Job drawing, mm, ordinate dimensions from the low corner. One solid piece. A direction names the side the tool comes from. Give positions to 0.01 mm unless a question says otherwise; leave off trailing zeros. Write each loop counter-clockwise with the first axis right and the second up, starting at its lowest first coordinate (ties: lowest second). Pieces come first, ordered by that corner, then holes. Notation, with made-up numbers: M 69.25,28 L 107.25,28 A19 cw 107.25,59 Z; hole C -31,14 d8. An arc over 180 degrees is marked long. Use CSV: the item, a comma, the result in double quotes. Start each with the question number.
Item 1: Pin check, flat tips, straight feed: pin 1 (2 mm diameter, centred on y = 1, z = 185, fed in from +X); pin 2 (6 mm diameter, centred on x = 156, z = 39, fed in from +Y); pin 3 (9 mm diameter, centred on x = 169.11, z = 295.93, fed in from +Y); pin 4 (4.5 mm diameter, centred on y = 2.5, z = 178, fed in from -X). Stop position of each tip, or through.
Item 2: Drill centre lines: line 1 (X direction, y = 15.5, z = 204); line 2 (Y direction, x = 129, z = 60); line 3 (X direction, y = 5, z = 231). Where is each one in solid material? Low to high. Write a range as [from, to].
Item 3: Cut at A-A (z = 315). List the corners of the cut face in (x, y), then the cut area to 3 significant figures.
Item 4: Cut at B-B (y = 17). List the corners of the cut face in (x, z), then the cut area to 3 significant figures.
Item 5: Which spindle directions (+Z, -Z, +X, -X, +Y, -Y) get a long thin tool onto all of the face, cutting with end or side? Do the marked faces 1 and 2. Say none if no direction does.
Item 6: Cut at D-D (x = 154.5). List the corners of the cut face in (y, z), then the cut area to 3 significant figures.
Item 7: Cut at C-C (z = 122). List the corners of the cut face in (x, y).
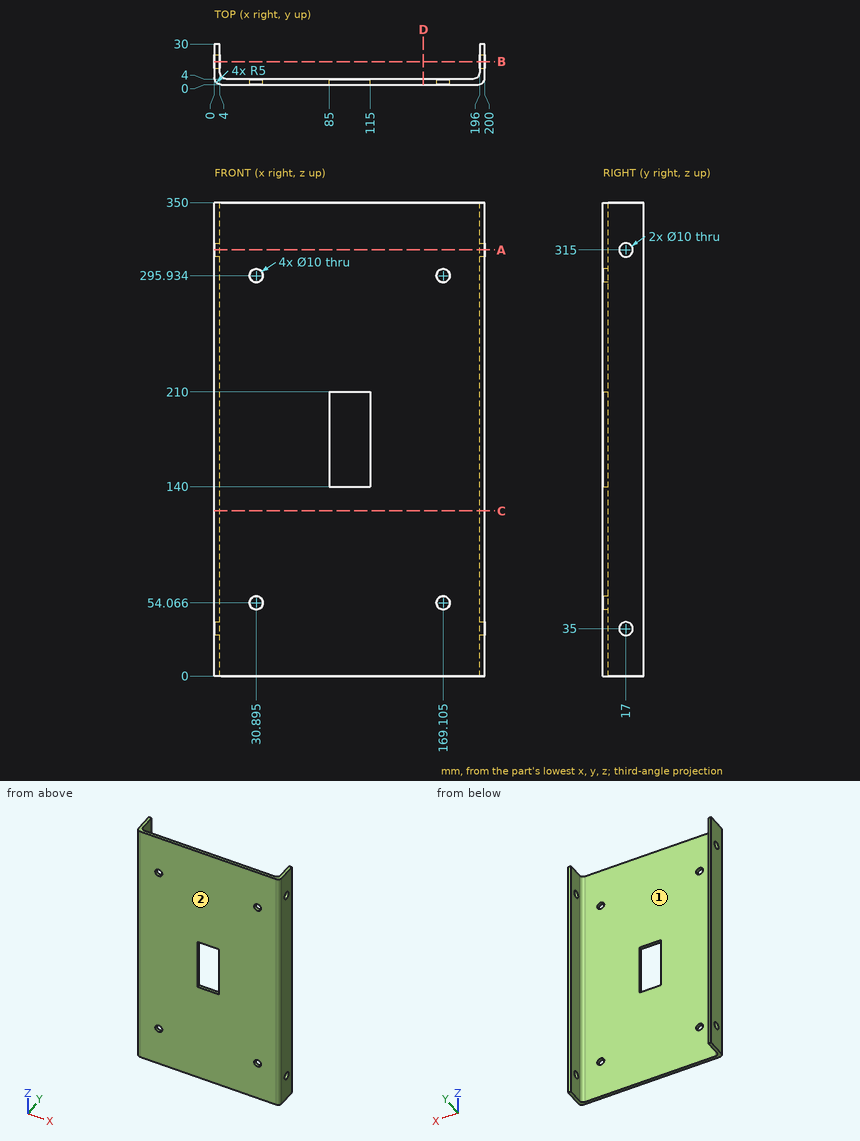
Worked answers:
1,pin 1,"stops at x = 199"
1,pin 2,"stops at y = 4"
1,pin 3,"passes through"
1,pin 4,"stops at x = 0.01"
2,line 1,"x = [0, 4], [196, 200]"
2,line 2,"y = [0, 4]"
2,line 3,"x = [0, 6], [194, 200]"
3,outline,"M 0,5 A5 ccw 5,0 L 195,0 A5 ccw 200,5 L 200,12 L 196,12 L 196,9 A5 cw 191,4 L 9,4 A5 cw 4,9 L 4,12 L 0,12 Z; M 0,22 L 4,22 L 4,30 L 0,30 Z; M 196,22 L 200,22 L 200,30 L 196,30 Z"
3,area,"928 mm^2"
4,outline,"M 0,0 L 4,0 L 4,30 L 0,30 Z; M 0,40 L 4,40 L 4,310 L 0,310 Z; M 0,320 L 4,320 L 4,350 L 0,350 Z; M 196,0 L 200,0 L 200,30 L 196,30 Z; M 196,40 L 200,40 L 200,310 L 196,310 Z; M 196,320 L 200,320 L 200,350 L 196,350 Z"
4,area,"2,640 mm^2"
5,face 1,"+Z, -Z, +Y"
5,face 2,"+Z, -Z, +X, -X, -Y"
6,outline,"M 0,0 L 4,0 L 4,350 L 0,350 Z"
6,area,"1,400 mm^2"
7,outline,"M 0,5 A5 ccw 5,0 L 195,0 A5 ccw 200,5 L 200,30 L 196,30 L 196,9 A5 cw 191,4 L 9,4 A5 cw 4,9 L 4,30 L 0,30 Z"
